```python
from build123d import *

# Parameters (mm, degrees)
SKETCH2_W                       = 152.4
SKETCH2_H                       = 12.7
SKETCH2_R                       = 4.7625
BOSS_EXTRUDE1_DEPTH             = 6.35
F_6_32_TAPPED_HOLE1_D           = 2.7051
F_6_32_TAPPED_HOLE1_CSINK_D     = 4.7752
F_6_32_TAPPED_HOLE1_CSINK_ANGLE = 90
F_6_32_TAPPED_HOLE2_D           = 2.7051
F_6_32_TAPPED_HOLE2_CSINK_D     = 4.7752
F_6_32_TAPPED_HOLE2_CSINK_ANGLE = 90


with BuildPart() as part:
    # Sketch2 → Boss-Extrude1 (new body)
    with BuildSketch(Plane.XY):
        Rectangle(SKETCH2_W, SKETCH2_H)
        with Locations((-63.5, 0)):
            Circle(SKETCH2_R, mode=Mode.SUBTRACT)
        with BuildLine():
            Line((0, -4.7625), (63.5, -4.7625))
            ThreePointArc((63.5, -4.7625), (68.2625, 0), (63.5, 4.7625))
            Line((63.5, 4.7625), (0, 4.7625))
            ThreePointArc((0, 4.7625), (-4.7625, 0), (0, -4.7625))
        make_face(mode=Mode.SUBTRACT)
    extrude(amount=BOSS_EXTRUDE1_DEPTH)

    # #6-32 Tapped Hole1 (through all)
    with Locations(Plane(origin=(0, 6.35, 0), x_dir=(1, 0, 0), z_dir=(0, 1, 0))):
        with Locations((-73.025, -3.175)):
            CounterSinkHole(F_6_32_TAPPED_HOLE1_D / 2, F_6_32_TAPPED_HOLE1_CSINK_D / 2, counter_sink_angle=F_6_32_TAPPED_HOLE1_CSINK_ANGLE)

    # #6-32 Tapped Hole2 (through all)
    with Locations(Plane(origin=(0, 6.35, 0), x_dir=(1, 0, 0), z_dir=(0, 1, 0))):
        with Locations((73.025, -3.175)):
            CounterSinkHole(F_6_32_TAPPED_HOLE2_D / 2, F_6_32_TAPPED_HOLE2_CSINK_D / 2, counter_sink_angle=F_6_32_TAPPED_HOLE2_CSINK_ANGLE)


solid = part.part
```
Input: part model. Units: mm. Frame: model coordinates. A direction names the side the tool comes from. Coordinates: 2 decimals unless noted, no trailing zeros. Write each loop counter-clockwise with the first axis right and the second up, starting at its lowest first coordinate (ties: lowest second). Pieces come first, ordered by that corner, then holes.
1) Section A-A on x = 5. Output: boundary loops of the cut face in (y, z).
2) Section B-B on y = 1.25. Output: boundary loops of the cut face in (x, z) (3 decimals), and give its area (3 significant figures).
3) Material intervals for line 1 along Y through (x, z) = (33, 1.75); line 2 along X through (y, z) = (4.25, 2.25); line 3 along X through (y, z) = (3.5, 3), sorted ascending.
4) Pin query (flat end, axial travel): pin 1 Ø3 at (x, z) = (73.025, 3.175) entering from -Y. Return the tip coordinate at first contact, or that it passes through.
5) Set-up query: faces 1 (the flat face through (76.2, 0, 3)), 2 (the flat face through (31, -4.762, 3)). Return all of +Z, -Z, +X, -X, +Y, -Y with unobstructed straight access to the full face (end or side cutting, diameter ignored); none if empty.
6) Mould query, pull axis Z, two halves, no side actions, for faces 3 (the flat face through (-18, 0, 0)), 4 (the flat face through (-1, -6.35, 3)), 5 (the cylindrical face through (-71.674, -0.599, 3.116)). Classes: pulls with the +Z half, pulls with the -Z half, needs draft (parallel to the pull), parting line crosses it, or undercut.
Check result:
1. outline: (-6.35, 0) - (-4.76, 0) - (-4.76, 6.35) - (-6.35, 6.35) - close; (4.76, 0) - (6.35, 0) - (6.35, 6.35) - (4.76, 6.35) - close
2. outline: (-76.2, 0) - (-68.096, 0) - (-68.096, 6.35) - (-76.2, 6.35) - close; (-58.904, 0) - (-4.596, 0) - (-4.596, 6.35) - (-58.904, 6.35) - close; (68.096, 0) - (76.2, 0) - (76.2, 6.35) - (68.096, 6.35) - close; hole circle Ø2.705 at (-73.025, 3.175); hole circle Ø2.705 at (73.025, 3.175)
2. area: 436 mm2
3. line 1: y = -6.35 to -4.76, 4.76 to 6.35
3. line 2: x = -76.2 to -74.01, -72.04 to -65.65, -61.35 to -2.15, 65.65 to 72.04, 74.01 to 76.2
3. line 3: x = -76.2 to -74.37, -71.68 to -66.73, -60.27 to -3.23, 66.73 to 71.68, 74.37 to 76.2
4. pin 1: stops at y = -6.35
5. face 1: +Z, -Z, +X, +Y, -Y
5. face 2: +Z, -Z
6. face 3: pulls with the -Z half
6. face 4: needs draft
6. face 5: undercut
